from build123d import *

# Parameters (mm, degrees)
BOSS_EXTRUDE2_DEPTH = 40
SKETCH3_R           = 3.1
SKETCH3_R_2         = 2.1
SKETCH3_R_3         = 2
CUT_EXTRUDE1_DEPTH  = 75.330343737
SKETCH4_R           = 2
CUT_EXTRUDE3_DEPTH  = 73.972597597


with BuildPart() as part:
    # Sketch1 → Boss-Extrude2 (new body)
    with BuildSketch(Plane(origin=(0, 0, 0), x_dir=(1, 0, 0), z_dir=(0, 1, 0))):
        Polygon((0, 0), (55, 0), (55, 5), (5, 5), (5, 35), (0, 35), align=None)
    extrude(amount=BOSS_EXTRUDE2_DEPTH)

    # Sketch3 → Cut-Extrude1 (cut, through all)
    with BuildSketch(Plane(origin=(0, 0, -5), x_dir=(-1, 0, 0), z_dir=(0, 0, -1))):
        with Locations((-40, 12)):
            Circle(SKETCH3_R)
        with Locations((-40, 23)):
            Circle(SKETCH3_R_2)
        with Locations((-49.2, 32)):
            Circle(SKETCH3_R_3)
        with Locations((-30.8, 32)):
            Circle(SKETCH3_R_3)
    extrude(amount=-CUT_EXTRUDE1_DEPTH, mode=Mode.SUBTRACT)

    # Sketch4 → Cut-Extrude3 (cut, through all)
    with BuildSketch(Plane(origin=(5, 0, 0), x_dir=(0, 0, -1), z_dir=(1, 0, 0))):
        with Locations((12, 32)):
            Circle(SKETCH4_R)
        with Locations((27, 20)):
            Circle(SKETCH4_R)
        with Locations((12, 8)):
            Circle(SKETCH4_R)
    extrude(amount=-CUT_EXTRUDE3_DEPTH, mode=Mode.SUBTRACT)


solid = part.part
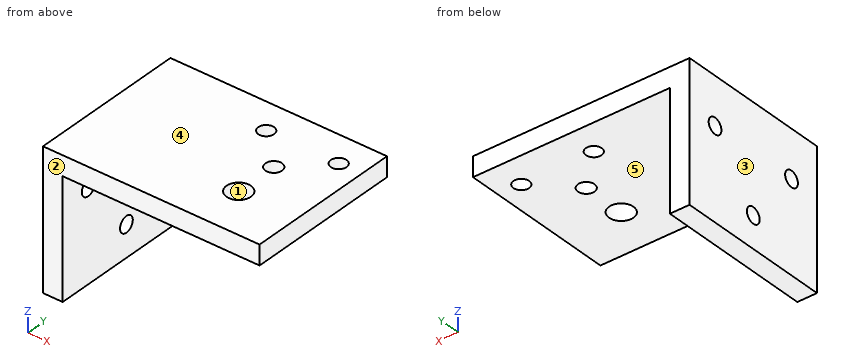
CAD build for the part. Positions are in the model's coordinates, mm. Face numbers are marked on the shaded views. A direction names the side the tool comes from. Give positions to 0.01 mm unless a question says otherwise; leave off trailing zeros. Order: outer loops, then holes, each group sorted by start corner. A loop starts at its lowest first (then second) coordinate and runs counter-clockwise, first axis right, second up. Notation, with made-up numbers: (24.25, -39) - (62.25, -39) arc R34 ccw to (62.25, -7) - close; hole circle Ø3 at (49.25, 22). An arc over 180 degrees is marked (long way). Answer in a Markdown table with one row per item.
1. Tool access for the marked faces 4 and 5: list every direction of +Z, -Z, +X, -X, +Y, -Y with a clear straight run to the whole face (end or side of a thin tool).
Data:
| item | result |
|---|---|
| face 4 | +Z, +X, -X, +Y, -Y |
| face 5 | -Z, +X, +Y, -Y |
2. Pull direction Y, two halves, no side cores. Call the marked faces 1, 2 and 3: pulls with the +Y half, pulls with the -Y half, needs draft (parallel to the pull), parting line crosses it, or undercut.
Data:
| item | result |
|---|---|
| face 1 | undercut |
| face 2 | pulls with the -Y half |
| face 3 | needs draft |
3. Flat gauge pins, fed straight in: pin 1 (10 mm diameter, centred on y = 15.5, z = -12, fed in from +X); pin 2 (3 mm diameter, centred on x = 49.2, y = 32, fed in from -Z); pin 3 (5 mm diameter, centred on x = 30.8, y = 32, fed in from -Z). Where does each tip first touch, or does it go through?
Data:
| item | result |
|---|---|
| pin 1 | stops at x = 5 |
| pin 2 | passes through |
| pin 3 | stops at z = -5 |
4. Saw through at A-A, the plane z = -27. Give the cut face in (x, y), plus the area to 3 significant figures.
Data:
| item | result |
|---|---|
| outline | (0, 0) - (5, 0) - (5, 18) - (0, 18) - close; (0, 22) - (5, 22) - (5, 40) - (0, 40) - close |
| area | 180 mm² |
5. Probe probe 1 along Y at (x, z) = (2, -12); probe 2 along Y at (x, z) = (40, -1.9); probe 3 along Y at (x, z) = (30.8, -3). List the from-to ranges inside material, lowest first. Write a range as [from, to].
Data:
| item | result |
|---|---|
| probe 1 | y = [0, 6], [10, 30], [34, 40] |
| probe 2 | y = [0, 8.9], [15.1, 20.9], [25.1, 40] |
| probe 3 | y = [0, 30], [34, 40] |
6. Saw through at B-B, the plane y = 12. Give the cut face in (x, z), plus the area to 3 significant figures.
Data:
| item | result |
|---|---|
| outline | (0, -35) - (5, -35) - (5, -5) - (36.9, -5) - (36.9, 0) - (0, 0) - close; (43.1, -5) - (55, -5) - (55, 0) - (43.1, 0) - close |
| area | 394 mm² |
7. Saw through at C-C, the plane x = 40. Give the cut face in (y, z), plus the area to 3 significant figures.
Data:
| item | result |
|---|---|
| outline | (0, -5) - (8.9, -5) - (8.9, 0) - (0, 0) - close; (15.1, -5) - (20.9, -5) - (20.9, 0) - (15.1, 0) - close; (25.1, -5) - (40, -5) - (40, 0) - (25.1, 0) - close |
| area | 148 mm² |
8. Saw through at D-D, the plane x = 30.8. Give the cut face in (y, z).
Data:
| item | result |
|---|---|
| outline | (0, -5) - (30, -5) - (30, 0) - (0, 0) - close; (34, -5) - (40, -5) - (40, 0) - (34, 0) - close |
